from build123d import *

# Parameters (mm, degrees)
SKETCH032_W     = 67
SKETCH032_H     = 84
PAD014_DEPTH    = 2
SKETCH033_R     = 1.25
POCKET_DEPTH    = 2.001
SKETCH034_R     = 2.5
PAD015_DEPTH    = 8
SKETCH035_R     = 2.5
PAD016_DEPTH    = 8
SKETCH036_R     = 1
POCKET009_DEPTH = 6
FILLET_R        = 2


with BuildPart() as part:
    # Sketch032 → Pad014 (new body)
    with BuildSketch(Plane.XY):
        with Locations((0, 10)):
            Rectangle(SKETCH032_W, SKETCH032_H)
    extrude(amount=PAD014_DEPTH)

    # Sketch033 (on Face6 of Pad014) → Pocket (cut, through all)
    with BuildSketch(Plane.XY.offset(2)):
        with Locations((-17.5, 36.5)):
            Circle(SKETCH033_R)
        with Locations((17.5, 36.5)):
            Circle(SKETCH033_R)
    extrude(amount=-POCKET_DEPTH, mode=Mode.SUBTRACT)

    # Sketch034 (on Face5 of Pocket) → Pad015 (join)
    with BuildSketch(Plane.XY.offset(2)):
        with Locations((-30.5, 49)):
            Circle(SKETCH034_R)
        with Locations((-30.5, -29)):
            Circle(SKETCH034_R)
        with Locations((30.5, 49)):
            Circle(SKETCH034_R)
        with Locations((30.5, -29)):
            Circle(SKETCH034_R)
    extrude(amount=PAD015_DEPTH)

    # Sketch035 (on Face5 of Pad015) → Pad016 (join)
    with BuildSketch(Plane.XY.offset(2)):
        with Locations((-24.5, 34)):
            Circle(SKETCH035_R)
        with Locations((24.5, 34)):
            Circle(SKETCH035_R)
        with Locations((-24.5, -24)):
            Circle(SKETCH035_R)
        with Locations((24.5, -24)):
            Circle(SKETCH035_R)
    extrude(amount=PAD016_DEPTH)

    # Sketch036 (on Face19 of Pad016) → Pocket009 (cut)
    with BuildSketch(Plane.XY.offset(10)):
        with Locations((-30.5, 49)):
            Circle(SKETCH036_R)
        with Locations((-24.5, 34)):
            Circle(SKETCH036_R)
        with Locations((30.5, 49)):
            Circle(SKETCH036_R)
        with Locations((24.5, 34)):
            Circle(SKETCH036_R)
        with Locations((30.5, -29)):
            Circle(SKETCH036_R)
        with Locations((24.5, -24)):
            Circle(SKETCH036_R)
        with Locations((-24.5, -24)):
            Circle(SKETCH036_R)
        with Locations((-30.5, -29)):
            Circle(SKETCH036_R)
    extrude(amount=-POCKET009_DEPTH, mode=Mode.SUBTRACT)

    # Fillet
    fillet_edges = [part.edges().sort_by_distance(p)[0] for p in [
        (-33.5, -32, 1),
        (33.5, -32, 1),
        (-33.5, 52, 1),
        (33.5, 52, 1),
    ]]
    fillet(fillet_edges, radius=FILLET_R)


with BuildPart() as part_1:
    # Body011 placement: moved
    add(part.part.moved(Location((0, 0, 3))))


solid = part_1.part
Geometry check sheet. Reference: the model listing, model coordinates, mm. A direction names the side the tool comes from. Round coordinates to 2 decimals unless told otherwise and drop trailing zeros. Loops run counter-clockwise (first coordinate to the right, second up) from the corner with the lowest first, then second, coordinate; pieces in that order, holes last.
Item 1: Cross-section at D-D on y = -29. Record the boundary of the cut face in (x, z).
Item 2: Cross-section at B-B on x = 17.5. Record the boundary of the cut face in (y, z).
Item 3: Mould release check, pull along Y, two halves, no side actions. Record for faces 3 (the flat face through (-33.5, 9, 4)), 4 (the cylindrical face through (-26, -22, 9)), 5 (the flat face through (0, -32, 4)): pulls with the +Y half, pulls with the -Y half, needs draft (parallel to the pull), parting line crosses it, or undercut.
Item 4: Gauge pin test, flat ends, axial feed: pin 1 (1.8 mm diameter, centred on x = 24.5, y = 34, fed in from +Z); pin 2 (5 mm diameter, centred on x = -11, y = -17, fed in from +Z). Record the tip position at first contact, or that the pin passes through.
Item 5: Cross-section at A-A on z = 11.75. Count the separate pieces of the cut face and the enclosed holes in it, then the cut area to 3 significant figures.
Item 6: Cross-section at C-C on x = -24.5. Record the boundary of the cut face in (y, z), then the cut area to 3 significant figures.
Item 7: Thickness scan on line 1 (Y direction, x = 30.5, z = 9.55); line 2 (Y direction, x = 24, z = 7.25); line 3 (Z direction, x = 20, y = -21.5). Record the ranges inside material, lowest first.
Item 8: Access from +Z, -Z, +X, -X, +Y, -Y to the whole of each face (thin tool, end or side, straight path). Record for faces 1 (the cylindrical face through (-24.63, 34.99, 10.04)), 2 (the cylindrical face through (18.655, 36.021, 4.014)).
Answer sheet:
1. outline: (-33.5, 3) - (33.5, 3) - (33.5, 5) - (33, 5) - (33, 13) - (31.5, 13) - (31.5, 7) - (29.5, 7) - (29.5, 13) - (28, 13) - (28, 5) - (-28, 5) - (-28, 13) - (-29.5, 13) - (-29.5, 7) - (-31.5, 7) - (-31.5, 13) - (-33, 13) - (-33, 5) - (-33.5, 5) - close
2. outline: (-32, 3) - (35.25, 3) - (35.25, 5) - (-32, 5) - close; (37.75, 3) - (52, 3) - (52, 5) - (37.75, 5) - close
3. face 3: needs draft
3. face 4: undercut
3. face 5: pulls with the -Y half
4. pin 1: stops at z = 7
4. pin 2: stops at z = 5
5. separate pieces: 8
5. enclosed holes: 8
5. area: 132 mm2
6. outline: (-32, 3) - (52, 3) - (52, 5) - (36.5, 5) - (36.5, 13) - (35, 13) - (35, 7) - (33, 7) - (33, 13) - (31.5, 13) - (31.5, 5) - (-21.5, 5) - (-21.5, 13) - (-23, 13) - (-23, 7) - (-25, 7) - (-25, 13) - (-26.5, 13) - (-26.5, 5) - (-32, 5) - close
6. area: 224 mm2
7. line 1: y = -31.5 to -30, -28 to -26.5, 46.5 to 48, 50 to 51.5
7. line 2: y = -26.45 to -24.87, -23.13 to -21.55, 31.55 to 33.13, 34.87 to 36.45
7. line 3: z = 3 to 5
8. face 1: +Z
8. face 2: +Z, -Z
